Read the model definition and answer for the solid it produces. Units are mm, in the model's axes. A direction names the side the tool comes from. Coordinates: 2 decimals unless noted, no trailing zeros. Loops run counter-clockwise (first coordinate to the right, second up) from the corner with the lowest first, then second, coordinate; pieces in that order, holes last. Notation, with made-up numbers: M -10,63.25 L 30,63.25 A35 ccw 30,100.25 Z; hole C -25.75,36.25 d10. An arc over 180 degrees is marked long. Use one line per item in the form item = value. Start each with the question number.
1. Find the intervals of material crossed by probe 1 along X at (y, z) = (6.5, -3.5); probe 2 along Y at (x, z) = (24.5, -4); probe 3 along X at (y, z) = (5, -6.25), in increasing order. Write a range as [from, to].
2. Flat-ended cylindrical pins translate along their axes: pin 1 (1 mm diameter, centred on y = 5, z = -0.5, fed in from +X); pin 2 (3 mm diameter, centred on x = 56, z = -6.5, fed in from +Y); pin 3 (4 mm diameter, centred on y = 87, z = 2.5, fed in from +X); pin 4 (12 mm diameter, centred on x = 61.5, y = 19.5, fed in from +Z). Find the tip coordinate at first contact, or state that the pin passes through.
3. For a pull along Z with two mould halves and no side action, classify faces 1 (the conical face through (2.29, 54.32, 2.99)), 2 (the cylindrical face through (66.335, 4.644, -0.071)), 3 (the flat face through (69, 6.2, 0.2)) as released by +Z, released by -Z, zero draft, split by the parting line, or undercut.
4. The part is cut by section B-B (y = 86). Give the vertices of the cut face in (x, z), plus the area to 3 significant figures.
5. The part is cut by section A-A (x = 46.5). Give the vertices of the cut face in (y, z), plus the area to 3 significant figures.
6. A tool of negligible diameter and unlimited length cuts with its end or side. For faces 4 (the flat face through (66, 5.472, 0)), 5 (the flat face through (42, 11, 0)), 6 (the flat face through (0, 0, 0)), 7 (the cylindrical face through (9.54, 7.44, -0.11)), from which of +Z, -Z, +X, -X, +Y, -Y can it reach the whole face along a straight path? Write none if from no direction.
7. The part is cut by section C-C (y = 41.5). Give the vertices of the cut face in (x, z).
from build123d import *

# Parameters (mm, degrees)
FILLET1_R           = 2.5
SKETCH2_R           = 2.443196487
BOSS_EXTRUDE1_DEPTH = 15
SKETCH3_W           = 26
SKETCH3_H           = 12
BOSS_EXTRUDE2_DEPTH = 54
FILLET2_R           = 1
CUT_EXTRUDE3_DEPTH  = 0.2
CUT_EXTRUDE4_DEPTH  = 5


with BuildPart() as part:
    # Sketch1 → Revolve1 (revolve)
    with BuildSketch(Plane.XY, mode=Mode.PRIVATE) as revolve1_sk:
        Polygon((0, 0), (0, 110), (2.5, 110), (5, 0), align=None)
    revolve(revolve1_sk.sketch.rotate(Axis((0, 0, 0), (0, 1, 0)), 90), axis=Axis((0, 0, 0), (0, 1, 0)))

    # Fillet1
    fillet1_edges = [part.edges().sort_by_distance(p)[0] for p in [
        (0, 110, 2.5),
        (0, 0, 5),
    ]]
    fillet(fillet1_edges, radius=FILLET1_R)

    # Sketch2 → Boss-Extrude1 (add)
    with BuildSketch(Plane(origin=(0, 0, 0), x_dir=(0, 0, -1), z_dir=(1, 0, 0))):
        with Locations(Location((0, 5, 0), (0, 0, 269.999999999))):
            Circle(SKETCH2_R)
    extrude(amount=BOSS_EXTRUDE1_DEPTH)

    # Sketch3 → Boss-Extrude2 (add)
    with BuildSketch(Plane(origin=(15, 0, 0), x_dir=(0, 0, -1), z_dir=(1, 0, 0))):
        with Locations((0, 5)):
            Rectangle(SKETCH3_W, SKETCH3_H)
    extrude(amount=BOSS_EXTRUDE2_DEPTH)

    # Fillet2
    fillet2_edges = [part.edges().sort_by_distance(p)[0] for p in [
        (15, 5, -13),
        (42, -1, -13),
        (15, 11, 0),
        (42, 11, -13),
        (15, 5, 13),
        (42, 11, 13),
        (15, -1, 0),
        (42, -1, 13),
        (69, 5, -13),
        (69, 11, 0),
        (69, 5, 13),
        (69, -1, 0),
    ]]
    fillet(fillet2_edges, radius=FILLET2_R)

    # Sketch6 → Cut-Extrude3 (cut)
    with BuildSketch(Plane(origin=(69, 0, 0), x_dir=(0, 0, -1), z_dir=(1, 0, 0))):
        with BuildLine():
            Line((-3.176393202, 6), (3.176393202, 6))
            ThreePointArc((3.176393202, 6), (3.346523364, 5.905146222), (3.35527864, 5.710557281))
            Line((3.35527864, 5.710557281), (2.55527864, 4.110557281))
            ThreePointArc((2.55527864, 4.110557281), (2.481539425, 4.029869838), (2.376393202, 4))
            Line((2.376393202, 4), (-2.376393202, 4))
            ThreePointArc((-2.376393202, 4), (-2.481539425, 4.029869838), (-2.55527864, 4.110557281))
            Line((-2.55527864, 4.110557281), (-3.35527864, 5.710557281))
            ThreePointArc((-3.35527864, 5.710557281), (-3.346523364, 5.905146222), (-3.176393202, 6))
        make_face()
    extrude(amount=-CUT_EXTRUDE3_DEPTH, mode=Mode.SUBTRACT)

    # Sketch8 → Cut-Extrude4 (cut)
    with BuildSketch(Plane(origin=(68.8, 0, 0), x_dir=(0, 0, -1), z_dir=(1, 0, 0))):
        with BuildLine():
            Line((0.047682537, 5.471989403), (1.485955512, 5.471989403))
            ThreePointArc((1.485955512, 5.471989403), (1.677632452, 5.32908538), (1.595395333, 5.104588908))
            ThreePointArc((1.595395333, 5.104588908), (0.047682537, 4.643562278), (-1.500030259, 5.104588908))
            ThreePointArc((-1.500030259, 5.104588908), (-1.582267378, 5.32908538), (-1.390590438, 5.471989403))
            Line((-1.390590438, 5.471989403), (0.047682537, 5.471989403))
        make_face()
    extrude(amount=-CUT_EXTRUDE4_DEPTH, mode=Mode.SUBTRACT)


solid = part.part
Computed values:
q1.probe_1 = [-3.36, 3.36], [15, 69]
q1.probe_2 = [-1, 11]
q1.probe_3 = [15, 69]
q2.pin_1 = 68.8
q2.pin_2 = 11
q2.pin_3 = 2.98
q2.pin_4 = through
q3.face_1 = split by the parting line
q3.face_2 = undercut
q3.face_3 = zero draft
q4.outline = C 0,0 d6.09
q4.area = 29.1 mm²
q5.outline = M -1,-12 A1 ccw 0,-13 L 10,-13 A1 ccw 11,-12 L 11,12 A1 ccw 10,13 L 0,13 A1 ccw -1,12 Z
q5.area = 311 mm²
q6.face_4 = +X
q6.face_5 = +Z, -Z, +X, +Y
q6.face_6 = +Z, -Z, -X, -Y
q6.face_7 = none
q7.outline = C 0,0 d8.11
